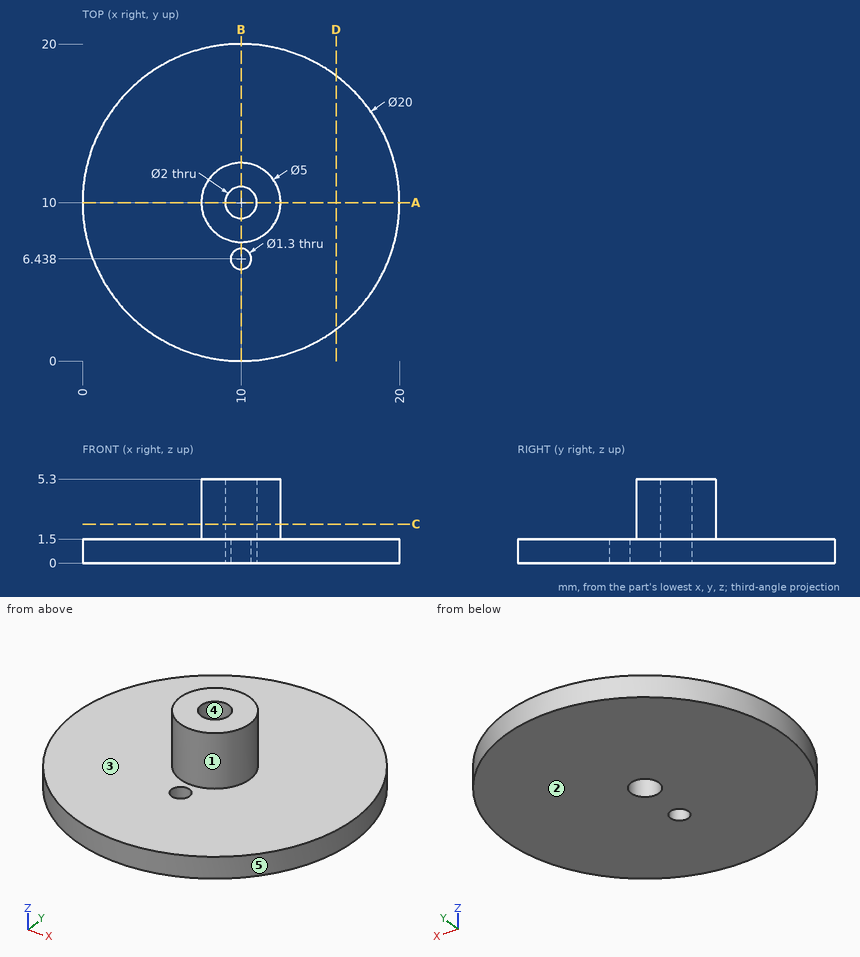
For this review, use the dimensioned drawing (mm, ordinates from the lowest corner) and the shaded views. A direction names the side the tool comes from. Coordinates: 2 decimals unless noted, no trailing zeros. Loops run counter-clockwise (first coordinate to the right, second up) from the corner with the lowest first, then second, coordinate; pieces in that order, holes last. Notation, with made-up numbers: (63.5, 71) -> (112.5, 71) arc R17 ccw to (112.5, 101) -> close; hole circle Ø4 at (-8.5, -24.75). An arc over 180 degrees is marked (long way). Return JSON: item names as keys, results as strings. Group by question number.
(1) Consider section A-A, the plane y = 10. Give the boundary of the cut face in (x, z), plus the area to 3 significant figures.
(2) Consider section C-C, the plane z = 2.45. Give the boundary of the cut face in (x, y).
(3) Tool access review of the marked faces 1 and 2: name each direction out of +Z, -Z, +X, -X, +Y, -Y from which nothing blocks a thin tool from reaching the whole face with its end or side.
(4) To check wall thickness, follow L1, parallel to Y at x = 10, z = 1.1; L2, parallel to Y at x = 10, z = 1.6; L3, parallel to Z at x = 17.25, y = 10. State the ranges of each line that lie inside material, in increasing order.
(5) For pin 1 Ø1.2 at (x, y) = (10, 10) entering from +Z; pin 2 Ø10 at (x, y) = (17.5, 7.5) entering from +Z; pin 3 Ø1 at (x, z) = (10, 2.5) entering from +Y, all flat-tipped, find the tip position at first contact; note any pin that passes through.
(6) Mouldability with a two-part tool opening along X and no side actions: class the marked faces 3, 4 and 5 as pulls with the +X half, pulls with the -X half, needs draft (parallel to the pull), parting line crosses it, or undercut.
(7) Consider section B-B, the plane x = 10. Give the boundary of the cut face in (y, z).
(8) Consider section D-D, the plane x = 16. Give the boundary of the cut face in (y, z), plus the area to 3 significant figures.
Results below:
{
 "1": {"outline": "(0, 0) -> (9, 0) -> (9, 5.3) -> (7.5, 5.3) -> (7.5, 1.5) -> (0, 1.5) -> close; (11, 0) -> (20, 0) -> (20, 1.5) -> (12.5, 1.5) -> (12.5, 5.3) -> (11, 5.3) -> close", "area": "38.4 mm2"},
 "2": {"outline": "circle Ø5 at (10, 10); hole circle Ø2 at (10, 10)"},
 "3": {"face 1": "+Z", "face 2": "-Z, +X, -X, +Y, -Y"},
 "4": {"L1": "y = 0 to 5.79, 7.09 to 9, 11 to 20", "L2": "y = 7.5 to 9, 11 to 12.5", "L3": "z = 0 to 1.5"},
 "5": {"pin 1": "passes through", "pin 2": "stops at z = 1.5", "pin 3": "stops at y = 12.5"},
 "6": {"face 3": "needs draft", "face 4": "undercut", "face 5": "parting line crosses it"},
 "7": {"outline": "(0, 0) -> (5.79, 0) -> (5.79, 1.5) -> (0, 1.5) -> close; (7.09, 0) -> (9, 0) -> (9, 5.3) -> (7.5, 5.3) -> (7.5, 1.5) -> (7.09, 1.5) -> close; (11, 0) -> (20, 0) -> (20, 1.5) -> (12.5, 1.5) -> (12.5, 5.3) -> (11, 5.3) -> close"},
 "8": {"outline": "(2, 0) -> (18, 0) -> (18, 1.5) -> (2, 1.5) -> close", "area": "24.0 mm2"}
}
